Autodesk Inventor part; units mm, degrees
ref_plane "YZ Plane" through (0, 0, 0) normal (1, 0, 0) x (0, 1, 0)
ref_plane "XZ Plane" through (0, 0, 0) normal (0, 1, 0) x (-1, 0, 0)
ref_plane "XY Plane" through (0, 0, 0) normal (0, 0, 1) x (1, 0, 0)
sketch "Sketch1" plane through (0, 0, 0) normal (0, 0, 1) x (1, 0, 0)
  line L0 (0, 0) -> (26.5, 0)
  line L1 (26.5, 0) -> (26.5, 51)
  line L2 (26.5, 51) -> (0, 51)
  line L3 (0, 51) -> (0, 0)
  line L4 (-3, 54) -> (29.5, 54)
  line L5 (29.5, 54) -> (29.5, -3)
  line L6 (29.5, -3) -> (-3, -3)
  line L7 (-3, -3) -> (-3, 54)
  line L8 (31.5, 56) -> (-5, 56)
  line L9 (-5, 56) -> (-5, -5)
  line L10 (-5, -5) -> (31.5, -5)
  line L11 (31.5, -5) -> (31.5, 56)
  line L12 (-3, 54) -> (-3, 56)
  line L13 (29.5, 54) -> (29.5, 56)
  line L14 (29.5, -3) -> (29.5, -5)
  line L15 (-3, -3) -> (-3, -5)
  dimension "d0" = 26.5
  dimension "d1" = 51
  dimension "d2" = 3
  dimension "d3" = 2
extrude "Extrusion1" add sketch "Sketch1" along normal blind 2 contours L3 L2 L1 L0 | L12 L8 L13 L4 | L4 L5 L6 L7 | L7 L15 L10 L9 L8 L12 | L13 L8 L11 L10 L14 L5 | L6 L14 L10 L15
extrude "Extrusion2" add sketch "Sketch1" along normal blind 24 contours L7 L15 L10 L9 L8 L12 | L13 L8 L11 L10 L14 L5
sketch "Sketch2" plane through (0, 0, 2) normal (0, 0, 1) x (1, 0, 0)
  line L0 (0, 0) -> (0, 51)
  line L1 (0, 25.5) -> (13.25, 25.5)
  line L2 (13.25, 25.5) -> (13.25, 49)
  line L3 (13.25, 49) -> (2.25, 49)
  circle A0 centre (2.25, 49) radius 1
  circle A1 centre (24.25, 49) radius 1
  circle A2 centre (2.25, 2) radius 1
  circle A3 centre (24.25, 2) radius 1
  circle A4 centre (2.25, 49) radius 2
  circle A5 centre (24.25, 49) radius 2
  circle A6 centre (2.25, 2) radius 2
  circle A7 centre (24.25, 2) radius 2
  dimension "d8" = 51
  dimension "d9" = 13.25
  dimension "d10" = 23.5
  dimension "d11" = 11
  dimension "d12" = 2
  dimension "d13" = 4
  dimension "d14" = 4
  dimension "d15" = 4
  dimension "d16" = 4
extrude "Extrusion3" add sketch "Sketch2" along normal blind 5
extrude "Extrusion4" cut sketch "Sketch2" against normal blind 5 contours A0 | A1 | A2 | A3
sketch "Sketch3" plane through (0, 0, 24) normal (0, 0, 1) x (1, 0, 0)
  line L0 (-5, 56) -> (-5, -5)
  line L1 (31.5, -5) -> (31.5, 56)
  line L2 (-5, -5) -> (31.5, -5)
  line L3 (31.5, -5) -> (31.5, 56)
  line L4 (31.5, 56) -> (-5, 56)
  line L5 (-5, 56) -> (-5, -5)
  point P0 (0, 0)
extrude "Extrusion5" add sketch "Sketch3" along normal blind 2
sketch "Sketch4" plane through (0, 0, 26) normal (0, 0, 1) x (1, 0, 0)
  line L0 (29.5, -5) -> (29.5, 56)
  line L1 (29.5, 56) -> (29.5, 51)
  line L2 (29.5, 51) -> (9.5, 51)
  line L3 (9.5, 51) -> (9.5, 41)
  line L4 (9.5, 41) -> (29.5, 41)
  line L5 (29.5, 41) -> (29.5, 51)
  line L6 (-3, 56) -> (-3, -5)
  line L7 (-3, -5) -> (-3, 0)
  line L8 (-3, 0) -> (17, 0)
  line L9 (17, 0) -> (17, 10)
  line L10 (17, 10) -> (-3, 10)
  line L11 (-3, 10) -> (-3, 0)
  point P0 (0, 0)
  dimension "d23" = 5
  dimension "d24" = 20
  dimension "d25" = 10
  dimension "d26" = 20
  dimension "d27" = 5
  dimension "d28" = 20
  dimension "d29" = 10
  dimension "d30" = 20
extrude "Extrusion6" cut sketch "Sketch4" against normal blind 2
sketch "Sketch5" plane through (0, 0, 26) normal (0, 0, 1) x (1, 0, 0)
  line L0 (-3, -5) -> (29.5, -5)
  line L1 (29.5, -5) -> (26.5, -5)
  line L2 (26.5, -5) -> (26.5, 15)
  line L3 (26.5, 15) -> (16.5, 15)
  line L4 (16.5, 15) -> (16.5, 30)
  line L5 (16.5, 30) -> (26.5, 30)
  line L6 (26.5, 30) -> (26.5, 15)
  circle A0 centre (24.25, 2) radius 2
  circle A1 centre (24.25, 2) radius 3
  circle A2 centre (2.25, 49) radius 1
  circle A3 centre (2.25, 49) radius 3
  point P0 (0, 0)
  dimension "d33" = 3
  dimension "d34" = 20
  dimension "d35" = 10
  dimension "d36" = 15
  dimension "d37" = 6
  dimension "d38" = 6
extrude "Extrusion7" cut sketch "Sketch5" against normal blind 2 contours A1 L2 | L3 L4 L5 L6 | L2 A1 | A0 | A2 | A3
sketch "Sketch6" plane through (31.5, -5, 0) normal (1, 0, 0) x (0, 0, -1)
  line L0 (-7, 5) -> (-7, 15)
  line L1 (-7, 15) -> (-20, 15)
  line L2 (-20, 15) -> (-20, 30)
  line L3 (-20, 30) -> (-7, 30)
  line L4 (-7, 30) -> (-7, 15)
  point P0 (0, 5)
  dimension "d41" = 10
  dimension "d42" = 13
  dimension "d43" = 15
extrude "Extrusion8" cut sketch "Sketch6" against normal blind 2
properties part number "case_dcdc_concerter"
Build history of the part. All positions in model axes, mm. A direction names the side the tool comes from. Coordinates: 2 decimals unless noted, no trailing zeros. Order: outer loops, then holes, each group sorted by start corner. A loop starts at its lowest first (then second) coordinate and runs counter-clockwise, first axis right, second up. Notation, with made-up numbers: (5.25, 65) - (12.25, 65) arc R29 cw to (12.25, 103) - close; hole circle Ø4 at (39, -35.75). An arc over 180 degrees is marked (long way). Put each result on its own line as item: value.
1. Probe line 1 along Y through (x, z) = (24.25, 25.2); line 2 along X through (y, z) = (2, 24.85); line 3 along Y through (x, z) = (24.25, 3.5). List the from-to ranges inside material, lowest first. Write a range as [from, to].
Answer sheet:
line 1: y = [-5, -1], [5, 15], [30, 41], [51, 56]
line 2: x = [-5, -3], [17, 21.25], [27.25, 31.5]
line 3: y = [0, 1], [3, 4], [47, 48], [50, 51]
2. Tool access for faces 4 (the face through (13, 26, 2)), 5 (the face through (31, 10, 13)), 6 (the face through (16.5, 22, 25)), 7 (the face through (13, 26, 24)): list every direction of +Z, -Z, +X, -X, +Y, -Y with a clear straight run to the whole face (end or side of a thin tool).
Answer sheet:
face 4: none
face 5: +X
face 6: +Z
face 7: +Y, -Y
3. Drop a flat-ended pin along its axis: P1, Ø3.5, axis at x = 24.25, y = 2, coming from the +Z side. Give the stop position or say it passes through.
Answer sheet:
P1: stops at z = 7
4. Pull direction X, two halves, no side cores. Call faces 1 (the face through (-5, 26, 13)), 2 (the face through (31, 18, 7)), 3 (the face through (7, 0, 25)): pulls with the +X half, pulls with the -X half, needs draft (parallel to the pull), parting line crosses it, or undercut.
Answer sheet:
face 1: pulls with the -X half
face 2: needs draft
face 3: undercut
5. Saw through at C-C (x = 18.5). Write the cut outline in (y, z).
Answer sheet:
outline: (-5, 0) - (56, 0) - (56, 2) - (-5, 2) - close; (-5, 24) - (15, 24) - (15, 26) - (-5, 26) - close; (30, 24) - (41, 24) - (41, 26) - (30, 26) - close; (51, 24) - (56, 24) - (56, 26) - (51, 26) - close
6. Saw through at A-A (z = 16.25). Write the cut outline in (x, y).
Answer sheet:
outline: (-5, -5) - (-3, -5) - (-3, 56) - (-5, 56) - close; (29.5, -5) - (31.5, -5) - (31.5, 10) - (29.5, 10) - close; (29.5, 25) - (31.5, 25) - (31.5, 56) - (29.5, 56) - close
7. Saw through at B-B (x = 2.25). Give the number of separate pieces and of enclosed holes in the cut face, and give its area (3 significant figures).
Answer sheet:
separate pieces: 6
enclosed holes: 0
area: 224 mm^2
